```python
from build123d import *

# Parameters (mm, degrees)
SKETCH1_R           = 5.1
SKETCH1_R_2         = 2
SKETCH1_R_3         = 3
BOSS_EXTRUDE1_DEPTH = 5


with BuildPart() as part:
    # Sketch1 → Boss-Extrude1 (new body)
    with BuildSketch(Plane(origin=(0, 0, 0), x_dir=(1, 0, 0), z_dir=(0, 1, 0))):
        with BuildLine():
            Line((-33.899726562, -8.414780986), (-9.506233548, -8.116743419))
            ThreePointArc((-9.506233548, -8.116743419), (12.499067121, 0.15271251), (-9.701705562, 7.882062496))
            Line((-9.701705562, 7.882062496), (-34.095198575, 7.584024929))
            ThreePointArc((-34.095198575, 7.584024929), (-49.996268483, -0.610850042), (-33.899726562, -8.414780986))
        make_face()
        with Locations((-20, 0)):
            Circle(SKETCH1_R, mode=Mode.SUBTRACT)
        with Locations((-3.1, 5.369357503)):
            Circle(SKETCH1_R_2, mode=Mode.SUBTRACT)
        with Locations((-3.1, -5.369357503)):
            Circle(SKETCH1_R_2, mode=Mode.SUBTRACT)
        Circle(SKETCH1_R_3, mode=Mode.SUBTRACT)
        with Locations((6.2, 0)):
            Circle(SKETCH1_R_2, mode=Mode.SUBTRACT)
    extrude(amount=BOSS_EXTRUDE1_DEPTH)


solid = part.part
```
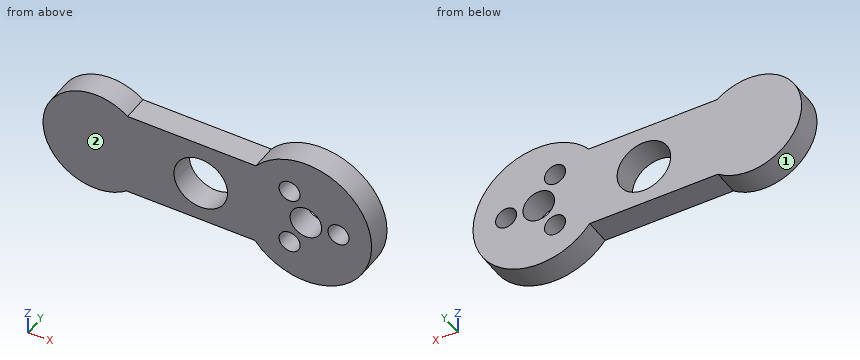
Geometry: final body of the model. Coordinates: model frame, mm. Face numbers are marked on the shaded views. Round coordinates to 2 decimals unless told otherwise and drop trailing zeros. Order: outer loops, then holes, each group sorted by start corner. A loop starts at its lowest first (then second) coordinate and runs counter-clockwise, first axis right, second up. Notation, with made-up numbers: M 55.5,6.25 L 75.5,6.25 A34 ccw 75.5,37.25 Z; hole C 23.25,-28.5 d8. An arc over 180 degrees is marked long. Use one line per item in the form item = value. Start each with the question number.
Q1. Material intervals for line 1 (X direction, y = 2.85, z = 0); line 2 (Z direction, x = -3.1, y = 2.3); line 3 (X direction, y = 2.75, z = 1), sorted ascending. Write a range as [from, to].
Q2. Cut plane D-D (y = 2.7). Return loops of the section in (x, z), and give its area (3 significant figures).
Q3. Mould query, pull axis X, two halves, no side actions, for the marked faces 1 and 2. Classes: +X half, -X half, draft (parallel to the pull), parting line (faces both ways), or undercut.
Q4. Cut plane C-C (z = -1.25). Return loops of the section in (x, y).
Q5. Pin query (flat end, axial travel): pin 1 Ø1 at (x, y) = (-42.5, 2) entering from -Z; pin 2 Ø1 at (y, z) = (1.5, -6.5) entering from -X; pin 3 Ø3 at (x, z) = (-3.1, -5.37) entering from +Y. Return the tip coordinate at first contact, or that it passes through.
Q6. Cut plane B-B (x = 6). Return loops of the section in (y, z), and give its area (3 significant figures).
Q7. Cut plane A-A (z = 6.75). Return loops of the section in (x, y), and give its area (3 significant figures).
Geometry results:
q1.line_1 = [-49.99, -25.1], [-14.9, -3], [3, 4.2], [8.2, 12.5]
q1.line_2 = [-12.11, -7.37], [-3.37, 3.37], [7.37, 12.11]
q1.line_3 = [-49.98, -25], [-15, -2.83], [2.83, 4.47], [7.93, 12.46]
q2.outline = M -34.1,-7.58 L -9.7,-7.88 A12.5 ccw long -9.51,8.12 L -33.9,8.41 A10 ccw long Z; hole C -20,0 d10.2; hole C -3.1,-5.37 d4; hole C -3.1,5.37 d4; hole C 0,0 d6; hole C 6.2,0 d4
q2.area = 971 mm^2
q3.face_1 = undercut
q3.face_2 = draft
q4.outline = M -49.84,0 L -24.94,0 L -24.94,5 L -49.84,5 Z; M -15.06,0 L -2.73,0 L -2.73,5 L -15.06,5 Z; M 2.73,0 L 4.64,0 L 4.64,5 L 2.73,5 Z; M 7.76,0 L 12.44,0 L 12.44,5 L 7.76,5 Z
q5.pin_1 = -9.31
q5.pin_2 = -47.61
q5.pin_3 = through
q6.outline = M 0,-10.97 L 5,-10.97 L 5,-1.99 L 0,-1.99 Z; M 0,1.99 L 5,1.99 L 5,10.97 L 0,10.97 Z
q6.area = 89.8 mm^2
q7.outline = M -47.79,0 L -4.55,0 L -4.55,5 L -47.79,5 Z; M -1.65,0 L 10.52,0 L 10.52,5 L -1.65,5 Z
q7.area = 277 mm^2
